Build history of the part. All positions in model axes, mm. A direction names the side the tool comes from. Round coordinates to 2 decimals unless told otherwise and drop trailing zeros. Write each loop counter-clockwise with the first axis right and the second up, starting at its lowest first coordinate (ties: lowest second). Pieces come first, ordered by that corner, then holes.
1) Saw through at D-D (z = -40). Write the cut outline in (x, y), plus the area to 3 significant figures.
2) Saw through at A-A (z = -18.5). Write the cut outline in (x, y), plus the area to 3 significant figures.
3) Wall check: probe 1 along Z at (x, y) = (-12.65, -12.8); probe 2 along Z at (x, y) = (-21.75, -3.8); probe 3 along X at (y, z) = (-9, -34). Give the ranges that are in metal, low to high.
4) Saw through at C-C (z = -31). Write the cut outline in (x, y), plus the area to 3 significant figures.
5) Saw through at B-B (x = 5). Write the cut outline in (y, z).
6) Pull direction Z, two halves, no side cores. Call faces 5 (the cylindrical face through (-13.19, -9.27, -8.11)), 6 (the flat face through (-14.2, -13, -38)), 7 (the flat face through (-1, -14, 0)), 8 (the cylindrical face through (-13.2, 2.7, -18.5)): +Z half, -Z half, draft (parallel to the pull), parting line (faces both ways), or undercut.
7) Which spindle directions (+Z, -Z, +X, -X, +Y, -Y) get a long thin tool onto all of the face, cutting with end or side? Do faces 1 (the cylindrical face through (-12.19, 0.54, 15.92)), 2 (the flat face through (-14.2, -11, -7)), 3 (the flat face through (8, 10, 0)), 4 (the cylindrical face through (-13.19, 4.72, -10.67)). Say none if no direction does.
8) Flat gauge pins, fed straight in: pin 1 (3.5 mm diameter, centred on y = 5.2, z = -40, fed in from -X); pin 2 (1 mm diameter, centred on y = -1, z = -27.5, fed in from +X); pin 3 (0.9 mm diameter, centred on y = 5.5, z = -40, fed in from -X). Where does each tip first touch, or does it go through?
from build123d import *

# Parameters (mm, degrees)
SKETCH1_R      = 12.2
EXTRUDE1_DEPTH = 32.3
SKETCH2_R      = 2.05
EXTRUDE2_DEPTH = 2.1
SKETCH3_R      = 6.75
EXTRUDE3_DEPTH = 4.6
SKETCH4_W      = 22.5
SKETCH4_H      = 32
EXTRUDE4_DEPTH = 46
SKETCH5_R      = 3.7
SKETCH5_R_2    = 1.5
SKETCH5_R_3    = 6.5
EXTRUDE5_DEPTH = 2
SKETCH6_R      = 3
EXTRUDE6_DEPTH = 14
SKETCH7_R      = 1.5
EXTRUDE7_DEPTH = 8


with BuildPart() as part:
    # Sketch1 → Extrude1 (new body)
    with BuildSketch(Plane.XY):
        Circle(SKETCH1_R)
    extrude(amount=EXTRUDE1_DEPTH)

    # Sketch2 → Extrude2 (add)
    with BuildSketch(Plane.XY.offset(32.3)):
        Circle(SKETCH2_R)
    extrude(amount=EXTRUDE2_DEPTH)

    # Sketch3 → Extrude3 (add)
    with BuildSketch(Plane.XY.offset(34.4)):
        Circle(SKETCH3_R)
    extrude(amount=EXTRUDE3_DEPTH)

    # Sketch4 → Extrude4 (add)
    with BuildSketch(Plane(origin=(0, 0, 0), x_dir=(-1, 0, 0), z_dir=(0, 0, -1))):
        with Locations((0.95, -3.8)):
            Rectangle(SKETCH4_W, SKETCH4_H)
    extrude(amount=EXTRUDE4_DEPTH)

    # Sketch5 → Extrude5 (add)
    # profile 1 of 6: a face of its own
    with BuildSketch(Plane.ZY.offset(12.2)):
        with Locations(Location((-40, -12.8, 0), (0, 0, 90))):
            Circle(SKETCH5_R)
        with Locations(Location((-40, -12.8, 0), (0, 0, 270))):
            Circle(SKETCH5_R_2, mode=Mode.SUBTRACT)
    # profile 2 of 6: a face of its own
    with BuildSketch(Plane.ZY.offset(12.2)):
        with Locations(Location((-40, 5.2, 0), (0, 0, 90))):
            Circle(SKETCH5_R)
        with Locations(Location((-40, 5.2, 0), (0, 0, 90))):
            Circle(SKETCH5_R_2, mode=Mode.SUBTRACT)
    # profile 3 of 6: a face of its own
    with BuildSketch(Plane.ZY.offset(12.2)):
        with Locations(Location((-7, 5.2, 0), (0, 0, 90))):
            Circle(SKETCH5_R)
        with Locations(Location((-7, 5.2, 0), (0, 0, 270))):
            Circle(SKETCH5_R_2, mode=Mode.SUBTRACT)
    # profile 4 of 6: a face of its own
    with BuildSketch(Plane.ZY.offset(12.2)):
        with Locations(Location((-7, -12.8, 0), (0, 0, 90))):
            Circle(SKETCH5_R)
        with Locations(Location((-7, -12.8, 0), (0, 0, 90))):
            Circle(SKETCH5_R_2, mode=Mode.SUBTRACT)
    # profile 5 of 6: a face of its own
    with BuildSketch(Plane.ZY.offset(12.2)):
        with Locations(Location((-31, -3.8, 0), (0, 0, 90))):
            Circle(SKETCH5_R_3)
    # profile 6 of 6: a face of its own
    with BuildSketch(Plane.ZY.offset(12.2)):
        with BuildLine():
            Line((-20, -8.8), (-20, 1.2))
            ThreePointArc((-20, 1.2), (-18.5, 2.7), (-17, 1.2))
            Line((-17, 1.2), (-17, -8.8))
            ThreePointArc((-17, -8.8), (-18.5, -10.3), (-20, -8.8))
        make_face()
    extrude(amount=EXTRUDE5_DEPTH)

    # Sketch6 → Extrude6 (add)
    with BuildSketch(Plane.ZY.offset(14.2)):
        with Locations(Location((-31, -3.8, 0), (0, 0, 270))):
            Circle(SKETCH6_R)
    extrude(amount=EXTRUDE6_DEPTH)

    # Sketch7 → Extrude7 (cut)
    with BuildSketch(Plane.ZY.offset(28.2)):
        with Locations(Location((-31, -3.8, 0), (0, 0, 270))):
            Circle(SKETCH7_R)
    extrude(amount=-EXTRUDE7_DEPTH, mode=Mode.SUBTRACT)


solid = part.part
Evaluation:
1. outline: (-14.2, -16.5) - (-12.2, -16.5) - (-12.2, -19.8) - (10.3, -19.8) - (10.3, 12.2) - (-12.2, 12.2) - (-12.2, 8.9) - (-14.2, 8.9) - (-14.2, 6.7) - (-12.2, 6.7) - (-12.2, 3.7) - (-14.2, 3.7) - (-14.2, 1.5) - (-12.2, 1.5) - (-12.2, -9.1) - (-14.2, -9.1) - (-14.2, -11.3) - (-12.2, -11.3) - (-12.2, -14.3) - (-14.2, -14.3) - close
1. area: 738 mm2
2. outline: (-14.2, -10.3) - (-12.2, -10.3) - (-12.2, -19.8) - (10.3, -19.8) - (10.3, 12.2) - (-12.2, 12.2) - (-12.2, 2.7) - (-14.2, 2.7) - close
2. area: 746 mm2
3. probe 1: z = -43.7 to -41.5, -38.5 to -36.3, -10.7 to -8.5, -5.5 to -3.3
3. probe 2: z = -34 to -32.5, -29.5 to -28
3. probe 3: x = -14.2 to 10.3
4. outline: (-28.2, -6.8) - (-14.2, -6.8) - (-14.2, -10.3) - (-12.2, -10.3) - (-12.2, -19.8) - (10.3, -19.8) - (10.3, 12.2) - (-12.2, 12.2) - (-12.2, 2.7) - (-14.2, 2.7) - (-14.2, -0.8) - (-28.2, -0.8) - (-28.2, -2.3) - (-20.2, -2.3) - (-20.2, -5.3) - (-28.2, -5.3) - close
4. area: 806 mm2
5. outline: (-19.8, -46) - (12.2, -46) - (12.2, 0) - (11.13, 0) - (11.13, 32.3) - (-11.13, 32.3) - (-11.13, 0) - (-19.8, 0) - close; (-4.53, 34.4) - (4.53, 34.4) - (4.53, 39) - (-4.53, 39) - close
6. face 5: undercut
6. face 6: draft
6. face 7: +Z half
6. face 8: undercut
7. face 1: +Z
7. face 2: +Z, -Z, -X, +Y, -Y
7. face 3: +Z, +X, +Y
7. face 4: -X
8. pin 1: stops at x = -14.2
8. pin 2: stops at x = 10.3
8. pin 3: stops at x = -12.2
